Geometry: final body of the model. Coordinates: model frame, mm. A direction names the side the tool comes from. Round coordinates to 2 decimals unless told otherwise and drop trailing zeros. Loops run counter-clockwise (first coordinate to the right, second up) from the corner with the lowest first, then second, coordinate; pieces in that order, holes last. Notation, with made-up numbers: (78, 34.5) - (83, 34.5) arc R20 cw to (83, 68.5) - close; hole circle Ø6 at (-9, -34.5). An arc over 180 degrees is marked (long way). Answer as a JSON object with one key per item and string values. Group by question number.
Item 1: Draft query along X for faces 4 (the face through (-20, 0.7, 24.1)), 5 (the face through (0, 0.7, 24.1)), 6 (the face through (10, 1, 17.5)), 7 (the face through (1, 0, 0)). Return one class per face: released by +X, released by -X, zero draft, split by the parting line, or undercut.
Item 2: Reachability of faces 1 (the face through (38.57, 0.74, -16)), 2 (the face through (-30, 1, 17.5)), 3 (the face through (-10, 2.457, 18)) from +Z, -Z, +X, -X, +Y, -Y: full face, straight path, thin tool, end or side. Return the list, or none.
Item 3: Line query: line 1 (Y direction, x = -3.75, z = 21.5); line 2 (Y direction, x = -17.5, z = 7); line 3 (Y direction, x = 25, z = 21). Output: solid intervals per line, ascending.
Item 4: Section D-D (z = -7.5). Return the cut outline in (x, y), plus the area to 3 significant figures.
Item 5: Section B-B (z = 5.5). Return the cut outline in (x, y), plus the area to 3 significant figures.
Item 6: First-contact query: pin 1 (0.8 mm diameter, centred on x = -34.5, y = 1, fed in from +Z); pin 2 (12 mm diameter, centred on x = 7.5, z = -12, fed in from -Y); pin 3 (3 mm diameter, centred on x = 25.5, z = -5.5, fed in from +Y). Flat tips, straight axial feed; report the tip coordinate or a pass-through.
Item 7: Section C-C (z = 21.5). Return the cut outline in (x, y), plus the area to 3 significant figures.
Item 8: Section A-A (x = -26). Return the cut outline in (y, z), plus the area to 3 significant figures.
```python
from build123d import *

# Parameters (mm, degrees)
BOSS_EXTRUDE1_DEPTH          = 1.5
BOSS_EXTRUDE2_DEPTH          = 20
LPATTERN1_COUNT              = 2
LPATTERN1_PITCH              = 40
CSK_FOR_M4_SFHCS1_AT_2_COUNT = 2
CSK_FOR_M4_SFHCS1_AT_2_PITCH = 29.068883707
CSK_FOR_M4_SFHCS1_AT_3_COUNT = 2
CSK_FOR_M4_SFHCS1_AT_3_PITCH = 52


with BuildPart() as part:
    # Sketch1 → Boss-Extrude1 (new body)
    with BuildSketch(Plane(origin=(0, 0, 0), x_dir=(1, 0, 0), z_dir=(0, 1, 0))):
        with BuildLine():
            Line((-40, -17.5), (40, -17.5))
            Line((40, -17.5), (40, 12.5))
            ThreePointArc((40, 12.5), (38.535533906, 16.035533906), (35, 17.5))
            Line((35, 17.5), (-35, 17.5))
            ThreePointArc((-35, 17.5), (-38.535533906, 16.035533906), (-40, 12.5))
            Line((-40, 12.5), (-40, -17.5))
        make_face()
    extrude(amount=BOSS_EXTRUDE1_DEPTH)

    # Sketch2 → Boss-Extrude2 (add)
    with BuildSketch(Plane(origin=(40, 0, 0), x_dir=(0, 0, -1), z_dir=(1, 0, 0))):
        with BuildLine():
            Line((-17.616081812, 2.45665015), (-19.190276967, 2.45665015))
            ThreePointArc((-19.190276967, 2.45665015), (-23.971620702, 1.124379043), (-19.010352011, 1.272727273))
            ThreePointArc((-19.010352011, 1.272727273), (-18.929937178, 1.434637236), (-18.761387212, 1.5))
            Line((-18.761387212, 1.5), (-17.5, 1.5))
            Line((-17.5, 1.5), (-17.5, 0))
            Line((-17.5, 0), (-17.627016654, 0))
            ThreePointArc((-17.627016654, 0), (-17.76259819, -0.039957987), (-17.854839204, -0.147058824))
            ThreePointArc((-17.854839204, -0.147058824), (-25.483287925, 1.865263339), (-17.616081812, 2.45665015))
        make_face()
    boss_extrude2 = extrude(amount=-BOSS_EXTRUDE2_DEPTH)

    # LPattern1: Boss-Extrude2 ×2
    with Locations(*[(-i * LPATTERN1_PITCH, 0, 0) for i in range(1, LPATTERN1_COUNT)]):
        add(boss_extrude2)

    # Sketch5 → CSK for M4 SFHCS1 (revolve, cut)
    with BuildSketch(Plane(origin=(-26, 1.5, 5.5), x_dir=(0, 0, 1), z_dir=(1, 0, 0))):
        Polygon((0, 0), (0, 4), (2.25, 4), (2.25, 2.23), (4.48, 0), align=None)
    csk_for_m4_sfhcs1 = revolve(axis=Axis((-26, 7.85, 5.5), (0, -1, 0)), mode=Mode.SUBTRACT)

    # CSK for M4 SFHCS1 at 2: CSK for M4 SFHCS1 ×2
    with Locations(*[Vector(0.894427190999916, 0, -0.44721359549995787) * (i * CSK_FOR_M4_SFHCS1_AT_2_PITCH) for i in range(1, CSK_FOR_M4_SFHCS1_AT_2_COUNT)]):
        add(csk_for_m4_sfhcs1, mode=Mode.SUBTRACT)

    # CSK for M4 SFHCS1 at 3: CSK for M4 SFHCS1 ×2
    with Locations(*[(i * CSK_FOR_M4_SFHCS1_AT_3_PITCH, 0, 0) for i in range(1, CSK_FOR_M4_SFHCS1_AT_3_COUNT)]):
        add(csk_for_m4_sfhcs1, mode=Mode.SUBTRACT)


solid = part.part
```
Values:
{
 "1": {"face 4": "released by -X", "face 5": "undercut", "face 6": "undercut", "face 7": "zero draft"},
 "2": {"face 1": "-Z, +X, +Y, -Y", "face 2": "+Z, -X, +Y, -Y", "face 3": "-Z, +X, -X"},
 "3": {"line 1": "y = -2.5 to -1, 4 to 5.5", "line 2": "y = 0 to 1.5", "line 3": "y = -2.47 to -0.95, 3.95 to 5.47"},
 "4": {"outline": "(-40, 0) - (-2.98, 0) - (-4.48, 1.5) - (-40, 1.5) - close; (2.98, 0) - (40, 0) - (40, 1.5) - (4.48, 1.5) - close", "area": "109 mm^2"},
 "5": {"outline": "(-40, 0) - (-28.98, 0) - (-30.48, 1.5) - (-40, 1.5) - close; (-23.02, 0) - (23.02, 0) - (21.52, 1.5) - (-21.52, 1.5) - close; (28.98, 0) - (40, 0) - (40, 1.5) - (30.48, 1.5) - close", "area": "97.6 mm^2"},
 "6": {"pin 1": "stops at z = 17.5", "pin 2": "stops at y = 0", "pin 3": "stops at y = 1.5"},
 "7": {"outline": "(-20, -2.5) - (0, -2.5) - (0, -1) - (-20, -1) - close; (-20, 4) - (0, 4) - (0, 5.5) - (-20, 5.5) - close; (20, -2.5) - (40, -2.5) - (40, -1) - (20, -1) - close; (20, 4) - (40, 4) - (40, 5.5) - (20, 5.5) - close", "area": "120 mm^2"},
 "8": {"outline": "(0, -17.5) - (1.5, -17.5) - (1.5, 1.02) - (0, 2.52) - close; (0, 8.48) - (1.5, 9.98) - (1.5, 17.5) - (0, 17.5) - close", "area": "41.3 mm^2"}
}
